Input: part model. Units: mm. Frame: model coordinates. A direction names the side the tool comes from. Coordinates: 2 decimals unless noted, no trailing zeros. Write each loop counter-clockwise with the first axis right and the second up, starting at its lowest first coordinate (ties: lowest second). Pieces come first, ordered by that corner, then holes. Notation, with made-up numbers: (-33, 37.5) - (-27, 37.5) arc R22 cw to (-27, 71.5) - close; hole circle Ø2 at (41, -23.75). An arc over 180 degrees is marked (long way). Use a Markdown table: item, result. Add a question column.
Q1. Material intervals for probe 1 along X at (y, z) = (-6, 2.5); probe 2 along Z at (x, y) = (18, -5.25) (1 decimal); probe 3 along Z at (x, y) = (-1.95, -13.18), sorted ascending. Write a range as from..to.
Q2. Pin query (flat end, axial travel): P1, Ø10, axis at x = 10, z = -10.5, coming from the -Y side; P2, Ø4, axis at x = 14.5, y = -10, coming from the +Z side; P3, Ø6, axis at x = 5.5, z = 14.5, coming from the -Y side. Return the tip coordinate at first contact, or that it passes through.
Q3. Mould query, pull axis Z, two halves, no side actions, for faces 5 (the face through (10, 1.27, -10)), 6 (the face through (-2.37, -14.535, -16.101)), 7 (the face through (10, -4, 1.588)). Classes: released by +Z, released by -Z, zero draft, split by the parting line, or undercut.
Q4. Set-up query: faces 1 (the face through (10.14, -0.79, 1.13)), 2 (the face through (-1.588, -13, -3)), 3 (the face through (10, -4, 3.175)), 4 (the face through (0, -4, 2)). Return all of +Z, -Z, +X, -X, +Y, -Y with unobstructed straight access to the full face (end or side cutting, diameter ignored); none if empty.
Q5. Section query B-B (z = -10). Give the number of separate pieces and of enclosed holes in the cut face, then the cut area to 3 significant figures.
Q6. Section query D-D (z = 20). Return the cut outline in (x, y) (1 decimal).
from build123d import *

# Parameters (mm, degrees)
SKETCH2_W                = 20
SKETCH2_H                = 20
BOSS_EXTRUDE1_DEPTH      = 1.27
HOLE1_OUTLINE_R          = 1.5
HOLE1_DEPTH              = 1.27
CONVERT_SOLID3_START     = -0.3175
CONVERT_SOLID3_OUTLINE_W = 20
CONVERT_SOLID3_OUTLINE_H = 20
CONVERT_SOLID3_OUTLINE_R = 1.5
CONVERT_SOLID3_DEPTH     = 0.3175
EDGE_FLANGE1_DEPTH       = 20
CUT_EXTRUDE1_REACH       = 40.263
SKETCH25_R               = 6.25
EDGE_FLANGE3_DEPTH       = 20
EDGE_FLANGE4_DEPTH       = 20
SKETCH31_R               = 1
BOSS_EXTRUDE2_DEPTH      = 1.5875
FILLET1_R                = 2


# Read off the part's stored shape, not the designer's step: Hole1, Convert-Solid3
# Sheet-metal steps are written as plain solids
with BuildPart() as part:
    # Sketch2 → Boss-Extrude1 (new body)
    with BuildSketch(Plane(origin=(0, 0, 0), x_dir=(1, 0, 0), z_dir=(0, 1, 0))):
        with Locations((10, 10)):
            Rectangle(SKETCH2_W, SKETCH2_H)
    extrude(amount=BOSS_EXTRUDE1_DEPTH)

    # Hole1 outline → Hole1 (cut)
    with BuildSketch(Plane(origin=(0, 0, 0), x_dir=(1, 0, 0), z_dir=(0, 1, 0))):
        with Locations((13, 10)):
            Circle(HOLE1_OUTLINE_R)
    extrude(amount=HOLE1_DEPTH, mode=Mode.SUBTRACT)

    # Convert-Solid3 outline → Convert-Solid3 (add)
    with BuildSketch(Plane(origin=(0, 0, 0), x_dir=(1, 0, 0), z_dir=(0, 1, 0)).offset(CONVERT_SOLID3_START)):
        with Locations((10, 10)):
            Rectangle(CONVERT_SOLID3_OUTLINE_W, CONVERT_SOLID3_OUTLINE_H)
        with Locations((13, 10)):
            Circle(CONVERT_SOLID3_OUTLINE_R, mode=Mode.SUBTRACT)
    extrude(amount=CONVERT_SOLID3_DEPTH)

    # Edge-Flange1 section (across the edge) → Edge-Flange1 (add)
    with BuildSketch(Plane(origin=(-1.5875, -0.3175, 0), x_dir=(1, 0, 0), z_dir=(0, 0, -1))):
        with BuildLine():
            Line((-1.5875, 1.5875), (-1.5875, 24.1375))
            Line((-1.5875, 24.1375), (0, 24.1375))
            Line((0, 24.1375), (0, 1.5875))
            ThreePointArc((0, 1.5875), (0.464967985, 0.464967985), (1.5875, 0))
            Line((1.5875, 0), (1.5875, -1.5875))
            ThreePointArc((1.5875, -1.5875), (-0.65756403, -0.65756403), (-1.5875, 1.5875))
        make_face()
    extrude(amount=EDGE_FLANGE1_DEPTH)

    # Sketch25 → Cut-Extrude1 (cut, up to next)
    with BuildSketch(Plane(origin=(-1.5875, 0, 0), x_dir=(0, 0, -1), z_dir=(1, 0, 0)), mode=Mode.PRIVATE) as cut_extrude1_sk1:
        with Locations(Location((10, -13.18, 0), (0, 0, 90))):
            Circle(SKETCH25_R)
    cut_extrude1_tool1 = extrude(cut_extrude1_sk1.sketch, amount=-CUT_EXTRUDE1_REACH, mode=Mode.PRIVATE) & part.part
    add(cut_extrude1_tool1.solids().sort_by_distance((-1.5875, -13.18, -10))[0], mode=Mode.SUBTRACT)

    # Edge-Flange3 section (across the edge) → Edge-Flange3 (add)
    with BuildSketch(Plane(origin=(20, -0.3175, 1.5875), x_dir=(0, 0, -1), z_dir=(-1, 0, 0))):
        with BuildLine():
            Line((-1.5875, 1.5875), (-1.5875, 5))
            Line((-1.5875, 5), (0, 5))
            Line((0, 5), (0, 1.5875))
            ThreePointArc((0, 1.5875), (0.464967985, 0.464967985), (1.5875, 0))
            Line((1.5875, 0), (1.5875, -1.5875))
            ThreePointArc((1.5875, -1.5875), (-0.65756403, -0.65756403), (-1.5875, 1.5875))
        make_face()
    extrude(amount=EDGE_FLANGE3_DEPTH)

    # Edge-Flange4 section (across the edge) → Edge-Flange4 (add)
    with BuildSketch(Plane(origin=(0, -6.905, 3.175), x_dir=(0, 1, 0), z_dir=(1, 0, 0))):
        with BuildLine():
            Line((-1.5875, 1.5875), (-1.5875, 1.6))
            Line((-1.5875, 1.6), (0, 1.6))
            Line((0, 1.6), (0, 1.5875))
            ThreePointArc((0, 1.5875), (0.464967985, 0.464967985), (1.5875, 0))
            Line((1.5875, 0), (1.5875, -1.5875))
            ThreePointArc((1.5875, -1.5875), (-0.65756403, -0.65756403), (-1.5875, 1.5875))
        make_face()
    extrude(amount=EDGE_FLANGE4_DEPTH)

    # Sketch31 → Boss-Extrude2 (add)
    with BuildSketch(Plane(origin=(0, -6.905, 0), x_dir=(1, 0, 0), z_dir=(0, 1, 0))):
        with BuildLine():
            Line((20, -4.775), (0, -4.775))
            Line((0, -4.775), (13.901931499, -23.029367025))
            ThreePointArc((13.901931499, -23.029367025), (19.927179344, -24.561576399), (22.7869765, -19.041355625))
            Line((22.7869765, -19.041355625), (20, -4.775))
        make_face()
        with Locations(Location((17.879736852, -20, 0), (0, 0, 270))):
            Circle(SKETCH31_R, mode=Mode.SUBTRACT)
    extrude(amount=-BOSS_EXTRUDE2_DEPTH)

    # Fillet1
    fillet1_edges = [part.edges().sort_by_distance(p)[0] for p in [
        (20, 0.47625, -20),
        (-2.38125, -24.455, 0),
        (-2.38125, -24.455, -20),
    ]]
    fillet(fillet1_edges, radius=FILLET1_R)


solid = part.part
Values follow:
| question | item | result |
|---|---|---|
| 1 | probe 1 | 0..20 |
| 1 | probe 2 | 1.6..3.2 |
| 1 | probe 3 | -20..-16.25, -3.75..0 |
| 2 | P1 | y = -0.32 |
| 2 | P2 | z = 24.55 |
| 2 | P3 | y = -8.49 |
| 3 | face 5 | zero draft |
| 3 | face 6 | undercut |
| 3 | face 7 | released by -Z |
| 4 | face 1 | -Z, +X, -X, -Y |
| 4 | face 2 | +Z, -Z, +X, -Y |
| 4 | face 3 | +Z, +X, -X, +Y |
| 4 | face 4 | +Z, -X, +Y, -Y |
| 5 | separate pieces | 3 |
| 5 | enclosed holes | 0 |
| 5 | area | 48.9 mm2 |
| 6 | outline | (11.6, -8.5) - (16.9, -8.5) - (16.9, -6.9) - (11.6, -6.9) - close; (18.9, -8.5) - (22.9, -8.5) - (22.9, -6.9) - (18.9, -6.9) - close |
